Build history of the part. All positions in model axes, mm. A direction names the side the tool comes from. Give positions to 0.01 mm unless a question says otherwise; leave off trailing zeros. Write each loop counter-clockwise with the first axis right and the second up, starting at its lowest first coordinate (ties: lowest second). Pieces come first, ordered by that corner, then holes. Notation, with made-up numbers: (-31.75, 84.5) -> (-13.75, 84.5) arc R11 cw to (-13.75, 96.5) -> close; hole circle Ø8 at (-26, 25.25). An arc over 180 degrees is marked (long way). Write item = value, one per line. Start each with the question number.
Q1. Saw through at A-A, the plane z = 0.5. List the corners of the cut face in (x, y).
Q2. Wall check: line 1 (Y direction, x = 0, z = 14.1); line 2 (X direction, y = 213, z = -12.75). Give the ranges that are in metal, low to high.
Q3. Saw through at B-B, the plane y = 383.5. List the corners of the cut face in (x, z).
Q4. Drop flat-ended pins along their axis: P1, Ø3.5, axis at x = 0, y = 70, coming from the +Z side; P2, Ø8, axis at x = 0, y = 340, coming from the +Z side. Give the stop position or say it passes through.
Q5. Tool access for faces 1 (the face through (14, 0, 0)), 2 (the face through (0, 218, -13)): list every direction of +Z, -Z, +X, -X, +Y, -Y with a clear straight run to the whole face (end or side of a thin tool).
from build123d import *

# Parameters (mm, degrees)
BOSS_EXTRUDE1_DEPTH = 430
SKETCH2_W           = 26
SKETCH2_H           = 26
CUT_EXTRUDE1_DEPTH  = 430
SKETCH3_R           = 3
CUT_EXTRUDE2_DEPTH  = 30


with BuildPart() as part:
    # Sketch1 → Boss-Extrude1 (new body)
    with BuildSketch(Plane(origin=(0, 0, 0), x_dir=(1, 0, 0), z_dir=(0, 1, 0))):
        Polygon((-15, 0), (-15, 15), (15, 15), (15, -15), (-15, -15), align=None)
    extrude(amount=BOSS_EXTRUDE1_DEPTH)

    # Sketch2 → Cut-Extrude1 (cut)
    with BuildSketch(Plane(origin=(0, 430, 0), x_dir=(1, 0, 0), z_dir=(0, 1, 0))):
        Rectangle(SKETCH2_W, SKETCH2_H)
    extrude(amount=-CUT_EXTRUDE1_DEPTH, mode=Mode.SUBTRACT)

    # Sketch3 → Cut-Extrude2 (cut)
    with BuildSketch(Plane.XY.offset(15)):
        with Locations((0, 360)):
            Circle(SKETCH3_R)
        with Locations((0, 340)):
            Circle(SKETCH3_R)
        with Locations((0, 90)):
            Circle(SKETCH3_R)
        with Locations((0, 70)):
            Circle(SKETCH3_R)
    extrude(amount=-CUT_EXTRUDE2_DEPTH, mode=Mode.SUBTRACT)


solid = part.part
Report:
q1.outline = (-15, 0) -> (-13, 0) -> (-13, 430) -> (-15, 430) -> close; (13, 0) -> (15, 0) -> (15, 430) -> (13, 430) -> close
q2.line_1 = 0 to 67, 73 to 87, 93 to 337, 343 to 357, 363 to 430
q2.line_2 = -15 to -13, 13 to 15
q3.outline = (-15, -15) -> (15, -15) -> (15, 15) -> (-15, 15) -> close; hole (-13, -13) -> (13, -13) -> (13, 13) -> (-13, 13) -> close
q4.P1 = through
q4.P2 = 15
q5.face_1 = +Z, -Z, +X, -X, -Y
q5.face_2 = +Y, -Y
